from build123d import *

# Parameters (mm, degrees)
SKETCH_R           = 3.75
SKETCH_R_2         = 1.5
SKETCH_R_3         = 1.55
SKETCH_W           = 15
SKETCH_H           = 10
PAD_DEPTH          = 4
SKETCH002_R        = 3
POCKET_DEPTH       = 3
CHAMFER001_SIZE    = 0.5
POCKET001_DEPTH    = 3
SKETCH003_W        = 7.5
SKETCH003_H        = 2.5
SKETCH003_H_2      = 1.75
PAD001_DEPTH       = 1
CHAMFER002_1_SIZE2 = 1.5
CHAMFER002_1_SIZE  = 0.8
CHAMFER002_2_SIZE2 = 1.5
CHAMFER002_2_SIZE  = 0.8
CHAMFER002_3_SIZE2 = 1.5
CHAMFER002_3_SIZE  = 0.8
CHAMFER002_4_SIZE2 = 1.5
CHAMFER002_4_SIZE  = 0.8
FILLET_R           = 1.5
FILLET001_R        = 1
FILLET002_R        = 5
FILLET003_R        = 2.5
CHAMFER003_SIZE    = 2


with BuildPart() as part:
    # Sketch → Pad (new body)
    with BuildSketch(Plane.YZ):
        with BuildLine():
            Line((0, 0), (105, 0))
            Line((105, 0), (105, 145))
            ThreePointArc((105, 145), (100.606602, 155.606602), (90, 160))
            Line((0, 160), (90, 160))
            Line((0, 160), (0, 0))
        make_face()
        with Locations((36, 90)):
            Circle(SKETCH_R, mode=Mode.SUBTRACT)
        with Locations((5, 155)):
            Circle(SKETCH_R_2, mode=Mode.SUBTRACT)
        with Locations((95, 150)):
            Circle(SKETCH_R_2, mode=Mode.SUBTRACT)
        with Locations((100, 5)):
            Circle(SKETCH_R_2, mode=Mode.SUBTRACT)
        with Locations((5, 5)):
            Circle(SKETCH_R_2, mode=Mode.SUBTRACT)
        with Locations((20.5, 105.5)):
            Circle(SKETCH_R_3, mode=Mode.SUBTRACT)
        with Locations((51.5, 105.5)):
            Circle(SKETCH_R_3, mode=Mode.SUBTRACT)
        with Locations((51.5, 74.5)):
            Circle(SKETCH_R_3, mode=Mode.SUBTRACT)
        with Locations((20.5, 74.5)):
            Circle(SKETCH_R_3, mode=Mode.SUBTRACT)
        with BuildLine():
            ThreePointArc((10, 26.55), (8.45, 25), (10, 23.45))
            Line((10, 23.45), (30, 23.45))
            ThreePointArc((30, 23.45), (31.55, 25), (30, 26.55))
            Line((10, 26.55), (30, 26.55))
        make_face(mode=Mode.SUBTRACT)
        with BuildLine():
            ThreePointArc((30, 17.5), (37.5, 25), (30, 32.5))
            Line((30, 32.5), (20.35156, 32.5))
            Line((32.022148, 64.5), (20.35156, 32.5))
            Line((48.941165, 64.5), (32.022148, 64.5))
            Line((89.97646, 10), (48.941165, 64.5))
            Line((12.145677, 10), (89.97646, 10))
            Line((14.880972, 17.5), (12.145677, 10))
            Line((30, 17.5), (14.880972, 17.5))
        make_face(mode=Mode.SUBTRACT)
        Polygon((61.458835, 64.5), (95, 64.5), (95, 19.95314), align=None, mode=Mode.SUBTRACT)
        with Locations((36, 110)):
            Rectangle(SKETCH_W, SKETCH_H, mode=Mode.SUBTRACT)
        with BuildLine():
            Line((14.516034, 150), (36.560478, 118))
            Line((48.5, 118), (36.560478, 118))
            Line((48.5, 118), (53.5, 130))
            Line((53.5, 130), (95, 130))
            Line((95, 130), (95, 142.5))
            ThreePointArc((87.5, 150), (89.696699, 144.696699), (95, 142.5))
            Line((14.516034, 150), (87.5, 150))
        make_face(mode=Mode.SUBTRACT)
    extrude(amount=PAD_DEPTH)

    # Sketch002 → Pocket (cut)
    with BuildSketch(Plane(origin=(0, 0, 0), x_dir=(0, 1, 0), z_dir=(-1, 0, 0))):
        with Locations((51.5, -105.5)):
            Circle(SKETCH002_R)
        with Locations((20.5, -105.5)):
            Circle(SKETCH002_R)
        with Locations((20.5, -74.5)):
            Circle(SKETCH002_R)
        with Locations((51.5, -74.5)):
            Circle(SKETCH002_R)
    extrude(amount=-POCKET_DEPTH, mode=Mode.SUBTRACT)

    # Chamfer001
    chamfer001_edges = [part.edges().sort_by_distance(p)[0] for p in [
        (0, 48.5, 105.5),
        (0, 17.5, 105.5),
        (0, 17.5, 74.5),
        (0, 48.5, 74.5),
    ]]
    chamfer(chamfer001_edges, length=CHAMFER001_SIZE)

    # Sketch001 → Pocket001 (cut)
    with BuildSketch(Plane(origin=(0, 0, 0), x_dir=(0, 1, 0), z_dir=(-1, 0, 0))):
        with BuildLine():
            Line((34.196597, -108.793538), (34.118854, -109.790511))
            Line((34.118854, -109.790511), (39.103722, -110.179223))
            Line((39.181464, -109.18225), (39.103722, -110.179223))
            ThreePointArc((50, -99.174484), (42.631213, -102.060099), (39.181464, -109.18225))
            Line((105, -99.174484), (50, -99.174484))
            Line((105, -99.174484), (105, -94.174484))
            Line((105, -94.174484), (50, -94.174484))
            ThreePointArc((50, -94.174484), (39.23589, -98.389707), (34.196597, -108.793538))
        make_face()
        Polygon((105, -124), (105, -120), (75, -120), (65, -118), (45, -118), (45, -126), (65, -126), (75, -124), align=None)
    extrude(amount=-POCKET001_DEPTH, mode=Mode.SUBTRACT)

    # Sketch003 (on Face1 of Pocket001) → Pad001 (join)
    with BuildSketch(Plane(origin=(0, 0, 0), x_dir=(0, 1, 0), z_dir=(-1, 0, 0))):
        with Locations((53.75, -95.424484)):
            Rectangle(SKETCH003_W, SKETCH003_H)
        with Locations((77.5, -97.924484)):
            Rectangle(SKETCH003_W, SKETCH003_H)
        with Locations((101.25, -95.424484)):
            Rectangle(SKETCH003_W, SKETCH003_H)
        with Locations((101.25, -120.875)):
            Rectangle(SKETCH003_W, SKETCH003_H_2)
        with Locations((78.75, -123.125)):
            Rectangle(SKETCH003_W, SKETCH003_H_2)
    extrude(amount=-PAD001_DEPTH)

    # Chamfer002 1
    chamfer002_1_edges = [part.edges().sort_by_distance(p)[0] for p in [
        (1, 101.25, 94.174484),
        (1, 53.75, 94.174484),
    ]]
    chamfer002_1_side = part.faces().sort_by_distance((1.6, 77.5, 94.174484))[0]
    chamfer(chamfer002_1_edges, length=CHAMFER002_1_SIZE, length2=CHAMFER002_1_SIZE2, reference=chamfer002_1_side)

    # Chamfer002 2
    chamfer002_2_edges = [part.edges().sort_by_distance(p)[0] for p in [
        (1, 77.5, 99.174484),
    ]]
    chamfer002_2_side = part.faces().sort_by_distance((1.547619, 77.5, 99.174484))[0]
    chamfer(chamfer002_2_edges, length=CHAMFER002_2_SIZE, length2=CHAMFER002_2_SIZE2, reference=chamfer002_2_side)

    # Chamfer002 3
    chamfer002_3_edges = [part.edges().sort_by_distance(p)[0] for p in [
        (1, 78.75, 124),
    ]]
    chamfer002_3_side = part.faces().sort_by_distance((1.590909, 91.022727, 124))[0]
    chamfer(chamfer002_3_edges, length=CHAMFER002_3_SIZE, length2=CHAMFER002_3_SIZE2, reference=chamfer002_3_side)

    # Chamfer002 4
    chamfer002_4_edges = [part.edges().sort_by_distance(p)[0] for p in [
        (1, 101.25, 120),
    ]]
    chamfer002_4_side = part.faces().sort_by_distance((1.590909, 88.977273, 120))[0]
    chamfer(chamfer002_4_edges, length=CHAMFER002_4_SIZE, length2=CHAMFER002_4_SIZE2, reference=chamfer002_4_side)

    # Fillet
    fillet_edges = [part.edges().sort_by_distance(p)[0] for p in [
        (2, 43.5, 105),
        (2, 43.5, 115),
        (2, 28.5, 105),
        (2, 28.5, 115),
    ]]
    fillet(fillet_edges, radius=FILLET_R)

    # Fillet001
    fillet001_edges = [part.edges().sort_by_distance(p)[0] for p in [
        (0.5, 75, 122.25),
        (0.5, 82.5, 122.25),
        (0.5, 97.5, 121.75),
        (0.5, 97.5, 96.674484),
        (0.5, 73.75, 96.674484),
        (0.5, 50, 96.674484),
        (0.5, 105, 96.674484),
        (0.5, 105, 121.75),
        (0.5, 81.25, 96.674484),
        (0.5, 57.5, 96.674484),
    ]]
    fillet(fillet001_edges, radius=FILLET001_R)

    # Fillet002
    fillet002_edges = [part.edges().sort_by_distance(p)[0] for p in [
        (2, 95, 130),
        (2, 53.5, 130),
        (3.5, 48.5, 118),
        (2, 36.560478, 118),
        (2, 95, 64.5),
        (2, 48.941165, 64.5),
        (2, 32.022148, 64.5),
        (2, 20.35156, 32.5),
    ]]
    fillet(fillet002_edges, radius=FILLET002_R)

    # Fillet003
    fillet003_edges = [part.edges().sort_by_distance(p)[0] for p in [
        (2, 61.458835, 64.5),
        (2, 14.880972, 17.5),
        (2, 12.145677, 10),
        (2, 95, 19.95314),
        (2, 89.97646, 10),
        (2, 14.516034, 150),
        (2, 95, 142.5),
        (2, 87.5, 150),
    ]]
    fillet(fillet003_edges, radius=FILLET003_R)

    # Chamfer003
    chamfer003_edges = [part.edges().sort_by_distance(p)[0] for p in [
        (0, 20, 26.55),
        (0, 98.5, 5),
        (0, 3.5, 5),
        (0, 3.5, 155),
        (0, 93.5, 150),
    ]]
    chamfer(chamfer003_edges, length=CHAMFER003_SIZE)


solid = part.part
The listing builds one solid part. Answer for the finished solid, in the listing's coordinates (mm). A direction names the side the tool comes from. Coordinates: 2 decimals unless noted, no trailing zeros. Write each loop counter-clockwise with the first axis right and the second up, starting at its lowest first coordinate (ties: lowest second). Pieces come first, ordered by that corner, then holes. Notation, with made-up numbers: (-12, -27) - (8, -27) arc R21 cw to (8, -20) - close; hole circle Ø1 at (-32.75, 43.25). An arc over 180 degrees is marked (long way). Return JSON: item names as keys, results as strings.
1. Consider line 1 along Y through (x, z) = (2.05, 74.5); line 2 along Z through (x, y) = (2.55, 5); line 3 along Y through (x, z) = (2.15, 110.5). Determine where each line is inside the solid, lowest interval first.
Final values:
{"line 1": "0 to 17.5, 23.5 to 48.5, 54.5 to 105", "line 2": "0 to 3.5, 6.5 to 153.5, 156.5 to 160", "line 3": "0 to 28.5, 43.5 to 105"}
2. The part is cut by section A-A on z = 74.5. Determine the outline of the cut face in (x, y), then the cut area to 3 significant figures.
Final values:
{"outline": "(0, 0) - (4, 0) - (4, 18.95) - (3, 18.95) - (3, 17.5) - (0.5, 17.5) - (0, 17) - close; (0, 24) - (0.5, 23.5) - (3, 23.5) - (3, 22.05) - (4, 22.05) - (4, 49.95) - (3, 49.95) - (3, 48.5) - (0.5, 48.5) - (0, 48) - close; (0, 55) - (0.5, 54.5) - (3, 54.5) - (3, 53.05) - (4, 53.05) - (4, 105) - (0, 105) - close", "area": "377 mm^2"}
3. For a pull along Y with two mould halves and no side action, classify faces 4 (the face through (1.97, 100.72, 155.49)), 5 (the face through (2, 52, 0)), 6 (the face through (2.028, 93.251, 25.045)) as +Y half, -Y half, draft (parallel to the pull), parting line (faces both ways), or undercut.
Final values:
{"face 4": "+Y half", "face 5": "draft", "face 6": "undercut"}
4. Which of the six approach directions +Z, -Z, +X, -X, +Y, -Y give full straight-line access (tool end or side, diameter ignored) to faces 1 (the face through (1.48, 40.85, 97.08)), 2 (the face through (2, 43.5, 110)), 3 (the face through (0, 52, 79))?
Final values:
{"face 1": "-X", "face 2": "+X, -X", "face 3": "+Z, -Z, -X, +Y, -Y"}
5. Each of these flat-tipped pins is pushed along its axis until it touches: pin 1 Ø1.5 at (x, z) = (1, 75) entering from -Y; pin 2 Ø0.8 at (x, z) = (0.5, 123.5) entering from +Y; pin 3 Ø5 at (y, z) = (95, 150) entering from -X; pin 4 Ø1.8 at (y, z) = (51, 106) entering from -X. Where does it stop, or does it pass through?
Final values:
{"pin 1": "y = 0", "pin 2": "y = 82.5", "pin 3": "x = 1", "pin 4": "x = 3"}
6. The part is cut by section B-B on z = 49. Determine the outline of the cut face in (x, y).
Final values:
{"outline": "(0, 0) - (4, 0) - (4, 26.37) - (0, 26.37) - close; (0, 60.61) - (4, 60.61) - (4, 73.13) - (0, 73.13) - close; (0, 95) - (4, 95) - (4, 105) - (0, 105) - close"}
